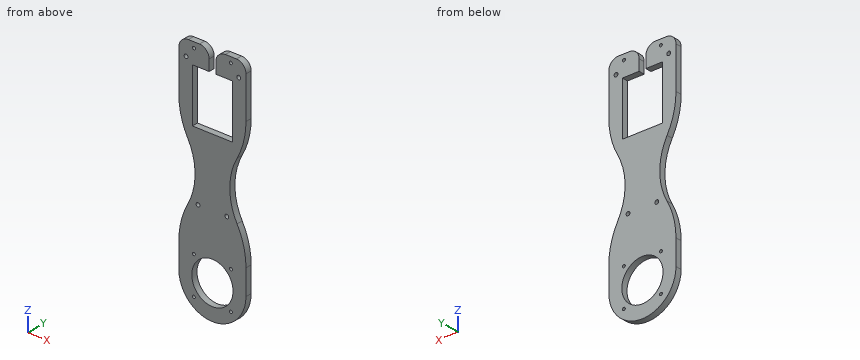
```python
from build123d import *

# Parameters (mm, degrees)
BOSS_EXTRUDE1_DEPTH = 3.175
SKETCH2_R           = 21.5
CUT_EXTRUDE1_DEPTH  = 215.322525648
SKETCH3_W           = 42
SKETCH3_H           = 55.35
SKETCH3_W_2         = 7
SKETCH3_H_2         = 21.35
CUT_EXTRUDE2_DEPTH  = 215.322525648
SKETCH4_R           = 1.5
CUT_EXTRUDE3_DEPTH  = 215.322525648
FILLET1_R           = 10
SKETCH5_R           = 2
CUT_EXTRUDE4_DEPTH  = 215.322525648
CUT_EXTRUDE5_DEPTH  = 215.322525648
FILLET3_R           = 76
SKETCH7_R           = 1.55
CUT_EXTRUDE6_DEPTH  = 215.322525648


with BuildPart() as part:
    # Sketch1 → Boss-Extrude1 (new, symmetric)
    with BuildSketch(Plane(origin=(0, 0, 0), x_dir=(1, 0, 0), z_dir=(0, 1, 0))):
        with BuildLine():
            Line((35, -211.35), (35, 0))
            ThreePointArc((35, 0), (0, 35), (-35, 0))
            Line((-35, 0), (-35, -211.35))
            Line((-35, -211.35), (35, -211.35))
        make_face()
    extrude(amount=BOSS_EXTRUDE1_DEPTH, both=True)

    # Sketch2 → Cut-Extrude1 (cut, through all)
    with BuildSketch(Plane(origin=(0, 3.175, 0), x_dir=(1, 0, 0), z_dir=(0, 1, 0))):
        with Locations(Location((0, 0, 0), (0, 0, 270))):
            Circle(SKETCH2_R)
    extrude(amount=-CUT_EXTRUDE1_DEPTH, mode=Mode.SUBTRACT)

    # Sketch3 → Cut-Extrude2 (cut, through all)
    with BuildSketch(Plane(origin=(0, 3.175, 0), x_dir=(1, 0, 0), z_dir=(0, 1, 0))):
        with Locations((0, -162.325)):
            Rectangle(SKETCH3_W, SKETCH3_H)
        with Locations((0, -200.675)):
            Rectangle(SKETCH3_W_2, SKETCH3_H_2)
    extrude(amount=-CUT_EXTRUDE2_DEPTH, mode=Mode.SUBTRACT)

    # Sketch4 → Cut-Extrude3 (cut, through all)
    with BuildSketch(Plane(origin=(0, 3.175, 0), x_dir=(1, 0, 0), z_dir=(0, 1, 0))):
        with Locations(Location((-19.35, 19.35, 0), (0, 0, 270))):
            Circle(SKETCH4_R)
        with Locations(Location((19.35, 19.35, 0), (0, 0, 270))):
            Circle(SKETCH4_R)
        with Locations(Location((19.35, -19.35, 0), (0, 0, 270))):
            Circle(SKETCH4_R)
        with Locations(Location((-19.35, -19.35, 0), (0, 0, 270))):
            Circle(SKETCH4_R)
    extrude(amount=-CUT_EXTRUDE3_DEPTH, mode=Mode.SUBTRACT)

    # Fillet1
    fillet1_edges = [part.edges().sort_by_distance(p)[0] for p in [
        (3.5, 0, 211.35),
        (-3.5, 0, 211.35),
        (35, 0, 211.35),
        (-35, 0, 211.35),
    ]]
    fillet(fillet1_edges, radius=FILLET1_R)

    # Sketch5 → Cut-Extrude4 (cut, through all)
    with BuildSketch(Plane(origin=(0, 3.175, 0), x_dir=(1, 0, 0), z_dir=(0, 1, 0))):
        with Locations(Location((-15, -65.35, 0), (0, 0, 270))):
            Circle(SKETCH5_R)
        with Locations(Location((15, -65.35, 0), (0, 0, 270))):
            Circle(SKETCH5_R)
        with Locations(Location((-27.5, -195.35, 0), (0, 0, 270))):
            Circle(SKETCH5_R)
        with Locations(Location((27.5, -195.35, 0), (0, 0, 270))):
            Circle(SKETCH5_R)
    extrude(amount=-CUT_EXTRUDE4_DEPTH, mode=Mode.SUBTRACT)

    # Sketch6 → Cut-Extrude5 (cut, through all)
    with BuildSketch(Plane.XZ.offset(3.175)):
        with BuildLine():
            Line((-35, 49.65), (-35, 134.65))
            ThreePointArc((-35, 134.65), (-18.102907984, 92.15), (-35, 49.65))
        make_face()
    cut_extrude5 = extrude(amount=-CUT_EXTRUDE5_DEPTH, mode=Mode.SUBTRACT)

    # Mirror1: Cut-Extrude5 across plane
    add(cut_extrude5.mirror(Plane(origin=(0, 0, 0), x_dir=(0, 0, 1), z_dir=(1, 0, 0))), mode=Mode.SUBTRACT)

    # Fillet3
    fillet3_edges = [part.edges().sort_by_distance(p)[0] for p in [
        (-35, 0, 134.65),
        (-35, 0, 49.65),
        (35, 0, 49.65),
        (35, 0, 134.65),
    ]]
    fillet(fillet3_edges, radius=FILLET3_R)

    # Sketch7 → Cut-Extrude6 (cut, through all)
    with BuildSketch(Plane.XZ.offset(3.175)):
        with Locations(Location((-19.25, 205.675, 0), (0, 0, 270))):
            Circle(SKETCH7_R)
        with Locations(Location((19.25, 205.675, 0), (0, 0, 270))):
            Circle(SKETCH7_R)
    extrude(amount=-CUT_EXTRUDE6_DEPTH, mode=Mode.SUBTRACT)


solid = part.part
```
Verification items for the finished model (mm, model axes). Give positions to 0.01 mm unless a question says otherwise; leave off trailing zeros. Loops run counter-clockwise (first coordinate to the right, second up) from the corner with the lowest first, then second, coordinate; pieces in that order, holes last.
1. Section check A-A, the plane x = 0. Enter the section's corners in (y, z) (3 decimals).
2. Section check C-C, the plane y = -1.75. Count the separate pieces of the cut face and the enclosed holes in it, then the cut area to 3 significant figures.
3. Section check D-D, the plane z = 57. Enter the section's corners in (x, y) (3 decimals), then the cut area to 3 significant figures.
4. Section check B-B, the plane z = -8. Enter the section's corners in (x, y) (3 decimals).
5. Thickness scan on line 1 (X direction, y = 1.5, z = 195.35); line 2 (X direction, y = -1.75, z = 197); line 3 (Z direction, x = -26, y = 1). Record the ranges inside material, lowest first.
6. Go/stop test with flat-tipped pins: pin 1 Ø1 at (x, y) = (10, -2.5) entering from +Z; pin 2 Ø3 at (x, y) = (21, -1) entering from -Z; pin 3 Ø3 at (y, z) = (1.5, 156.5) entering from -X. Record where each tip stops, or that it passes through.
Geometry says:
1. outline: (-3.175, -35) - (3.175, -35) - (3.175, -21.5) - (-3.175, -21.5) - close; (-3.175, 21.5) - (3.175, 21.5) - (3.175, 134.65) - (-3.175, 134.65) - close
2. separate pieces: 1
2. enclosed holes: 11
2. area: 10,500 mm2
3. outline: (-28.394, -3.175) - (28.394, -3.175) - (28.394, 3.175) - (-28.394, 3.175) - close
3. area: 361 mm2
4. outline: (-34.073, -3.175) - (-19.956, -3.175) - (-19.956, 3.175) - (-34.073, 3.175) - close; (19.956, -3.175) - (34.073, -3.175) - (34.073, 3.175) - (19.956, 3.175) - close
5. line 1: x = -35 to -29.5, -25.5 to -3.5, 3.5 to 25.5, 29.5 to 35
5. line 2: x = -35 to -28.63, -26.37 to -3.5, 3.5 to 26.37, 28.63 to 35
5. line 3: z = -23.43 to 61.88, 122.42 to 194.03, 196.67 to 211.3
6. pin 1: stops at z = 210.89
6. pin 2: stops at z = -29.06
6. pin 3: stops at x = -35
